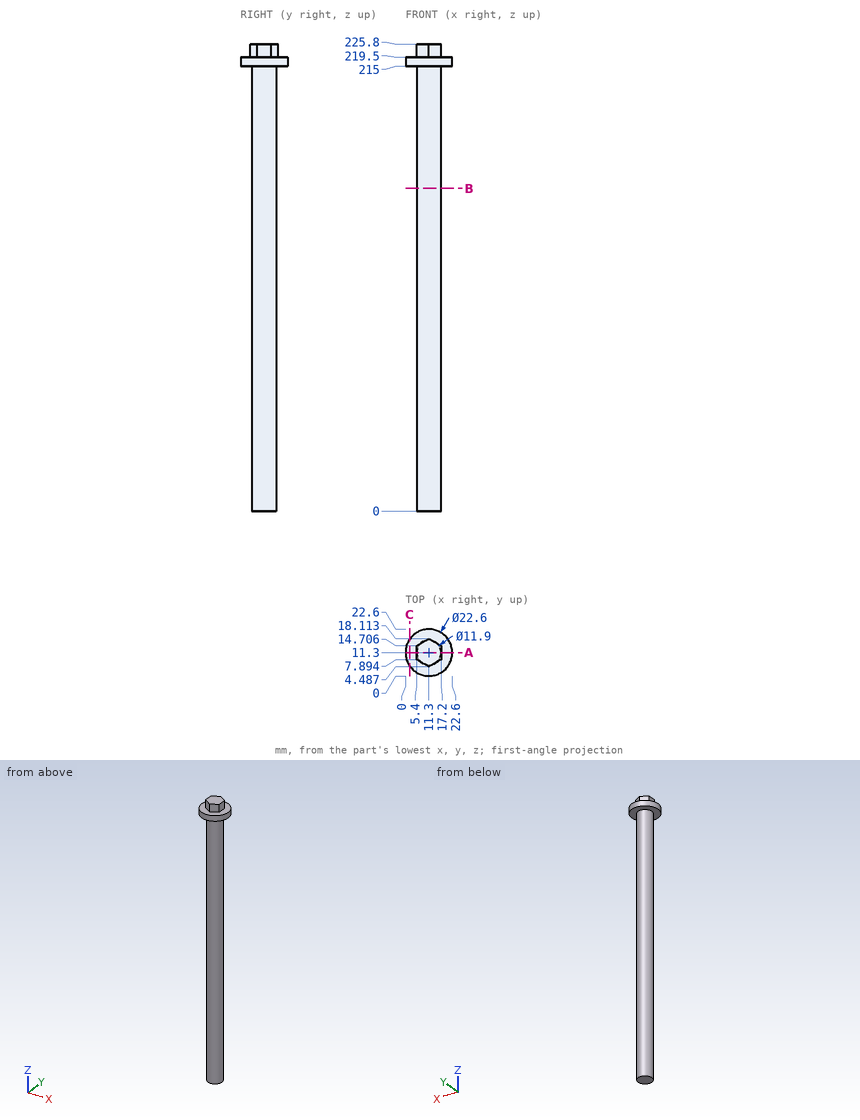
Geometry check sheet. Reference: drawing and pictorial views, mm from the part's lowest x, y, z. Coordinates: 2 decimals unless noted, no trailing zeros. Write each loop counter-clockwise with the first axis right and the second up, starting at its lowest first coordinate (ties: lowest second). Pieces come first, ordered by that corner, then holes. Notation, with made-up numbers: (-31, 8) -> (-19, 8) arc R16 ccw to (-19, 16) -> close; hole circle Ø8 at (59, 45.25). An arc over 180 degrees is marked (long way). One line per question, with ' | ' between items.
1. Thickness scan on probe 1 along Y at (x, z) = (11.75, 128); probe 2 along Z at (x, y) = (13, 2.75); probe 3 along Y at (x, z) = (8, 159). Record the ranges inside material, lowest first. Write a range as from..to.
Answers:
probe 1: y = 5.37..17.23 | probe 2: z = 215..219.5 | probe 3: y = 6.35..16.25
2. Cross-section at B-B on z = 156. Record the cut outline in (x, y), and give its area (3 significant figures).
Answers:
outline: circle Ø11.9 at (11.3, 11.3) | area: 111 mm²
3. Cross-section at A-A on y = 11.3. Record the cut outline in (x, z).
Answers:
outline: (0, 215) -> (5.35, 215) -> (5.35, 0) -> (17.25, 0) -> (17.25, 215) -> (22.6, 215) -> (22.6, 219.5) -> (17.2, 219.5) -> (17.2, 225.8) -> (5.4, 225.8) -> (5.4, 219.5) -> (0, 219.5) -> close
4. Cross-section at C-C on x = 2. Record the cut outline in (y, z).
Answers:
outline: (4.88, 215) -> (17.72, 215) -> (17.72, 219.5) -> (4.88, 219.5) -> close
5. Depth check by flat-ended pin: pin 1 Ø3 at (x, y) = (19, 15) entering from +Z; pin 2 Ø3 at (y, z) = (10.5, 224) entering from +X; pin 3 Ø1.5 at (x, z) = (16, 168) entering from -Y. Enter the tip coordinate at first touch or a pass-through.
Answers:
pin 1: stops at z = 219.5 | pin 2: stops at x = 17.2 | pin 3: stops at y = 6.85
